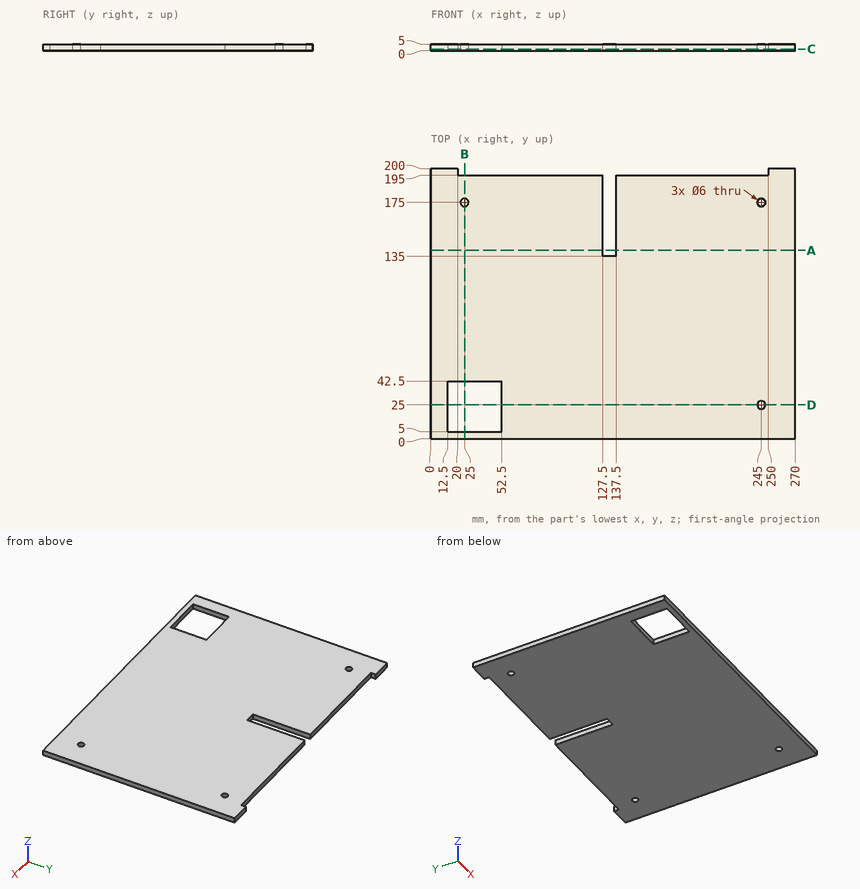
Design review of the part shown in the three views and the two pictorial views. Dimensions are in mm from the part's minimum x, y and z. Round coordinates to 2 decimals unless told otherwise and drop trailing zeros. Loops run counter-clockwise (first coordinate to the right, second up) from the corner with the lowest first, then second, coordinate; pieces in that order, holes last. Notation, with made-up numbers: (-34, -11) -> (-3, -11) arc R15 cw to (-3, -6) -> close; hole circle Ø3 at (-32, 0). An arc over 180 degrees is marked (long way). Answer as CSV lines item,"result".
1) To check wall thickness, follow line 1 along Y through (x, z) = (245, 2.95); line 2 along X through (y, z) = (175, 1.8); line 3 along X through (y, z) = (160.5, 4.2). State the ranges of each line that lie inside material, in increasing order. Write a range as from..to.
Geometry results:
line 1,"y = 0..22, 28..172, 178..195"
line 2,"x = 0..22, 28..127.5, 137.5..242, 248..270"
line 3,"x = 0..127.5, 137.5..270"
2) For P1, Ø2, axis at x = 172.5, z = 2, coming from the +Y side; P2, Ø5.5, axis at x = 25, y = 175, coming from the -Z side, all flat-tipped, find the tip position at first contact; note any pin that passes through.
Geometry results:
P1,"stops at y = 195"
P2,"passes through"
3) Add section A-A on y = 139.5. Write out the cut boundary in (x, z).
Geometry results:
outline,"(0, 0) -> (127.5, 0) -> (127.5, 5) -> (0, 5) -> close; (137.5, 0) -> (270, 0) -> (270, 5) -> (137.5, 5) -> close"
4) Add section D-D on y = 25. Write out the cut boundary in (x, z).
Geometry results:
outline,"(0, 0) -> (12.5, 0) -> (12.5, 5) -> (0, 5) -> close; (52.5, 0) -> (242, 0) -> (242, 5) -> (52.5, 5) -> close; (248, 0) -> (270, 0) -> (270, 5) -> (248, 5) -> close"
5) Add section B-B on x = 25. Write out the cut boundary in (y, z).
Geometry results:
outline,"(0, 0) -> (5, 0) -> (5, 5) -> (0, 5) -> close; (42.5, 0) -> (172, 0) -> (172, 5) -> (42.5, 5) -> close; (178, 0) -> (195, 0) -> (195, 5) -> (178, 5) -> close"
6) Add section C-C on z = 1.25. Write out the cut boundary in (x, y).
Geometry results:
outline,"(0, 0) -> (270, 0) -> (270, 200) -> (250, 200) -> (250, 195) -> (137.5, 195) -> (137.5, 135) -> (127.5, 135) -> (127.5, 195) -> (20, 195) -> (20, 200) -> (0, 200) -> close; hole (12.5, 5) -> (52.5, 5) -> (52.5, 42.5) -> (12.5, 42.5) -> close; hole circle Ø6 at (25, 175); hole circle Ø6 at (245, 25); hole circle Ø6 at (245, 175)"
